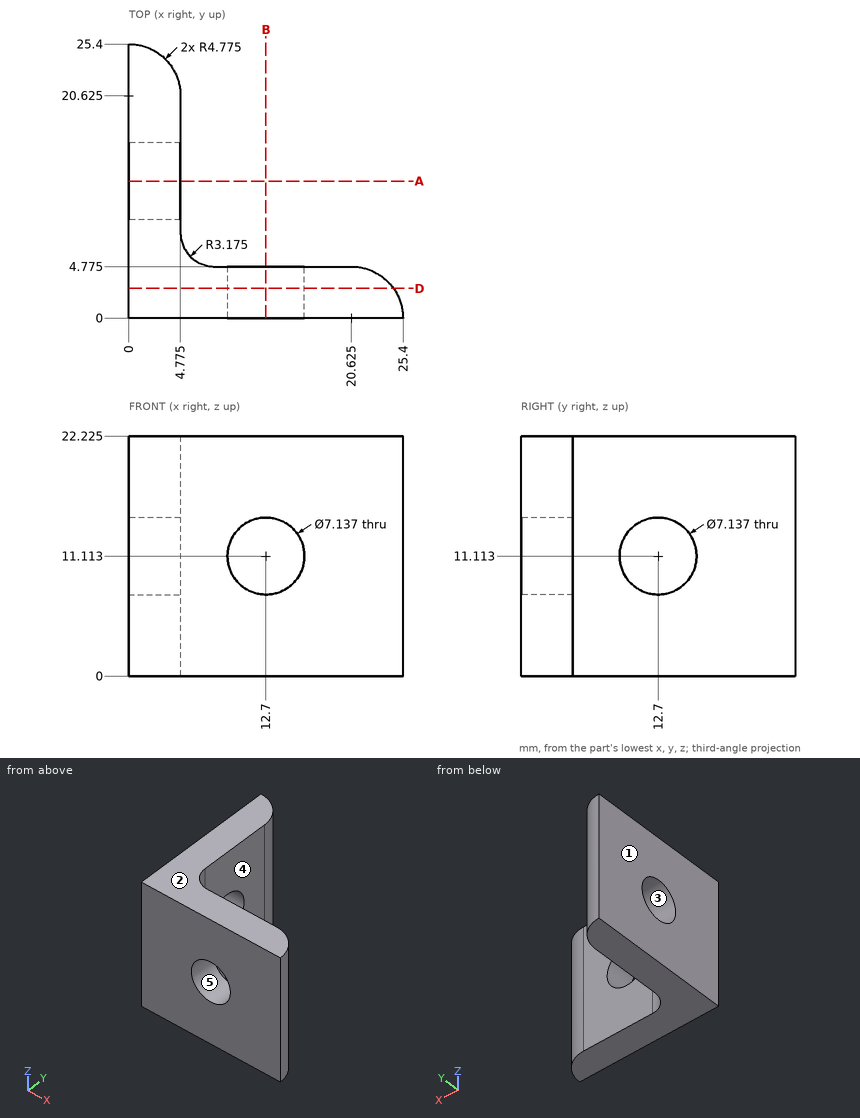
The drawing under review shows one solid part. Ordinate dimensions are in mm from its lowest x, y, z. A direction names the side the tool comes from. Round coordinates to 2 decimals unless told otherwise and drop trailing zeros. Loops run counter-clockwise (first coordinate to the right, second up) from the corner with the lowest first, then second, coordinate; pieces in that order, holes last. Notation, with made-up numbers: (16, -16) - (27, -16) arc R26 ccw to (27, 2) - close; hole circle Ø8 at (83, -19.5). An arc over 180 degrees is marked (long way). Use a Markdown table: item, result. Add a question column.
Q1. Add section D-D (y = 2.75). State the section outline as (x, z) points (1 decimal), plus the area to 3 significant figures.
Q2. The part is to be moulded in two halves that separate along Z. For the marked faces 1, 2 and 3, say which applies: pulls with the +Z half, pulls with the -Z half, needs draft (parallel to the pull), parting line crosses it, or undercut.
Q3. Machinability: for the marked faces 4 and 5, which of the approach directions +Z, -Z, +X, -X, +Y, -Y give a long, thin tool a straight path to every point of the face, cutting with its end or side? Answer none if there is none.
Q4. Add section A-A (y = 12.7). State the section outline as (x, z) points (1 decimal).
Q5. For probe 1 along Y at (x, z) = (18, 9.75) (1 decimal); probe 2 along Z at (x, y) = (3.7, 12.7) (1 decimal), list the stretches that pass through material, from the lowest coordinate up.
Q6. Insertion check: pin 1 Ø4.5 at (y, z) = (12.7, 11.11) entering from +X; pin 2 Ø10 at (x, z) = (16, 9.5) entering from +Y (1 decimal); pin 3 Ø5 at (y, z) = (8.5, 17) entering from +X (1 decimal); pin 4 Ø8 at (y, z) = (15.5, 14) entering from +X (1 decimal). Each pin has a flat end and moves straight along its axis. Give the tip position at first contact, or say it passes through.
Worked answers:
| question | item | result |
|---|---|---|
| 1 | outline | (0, 0) - (24.5, 0) - (24.5, 22.2) - (0, 22.2) - close; hole circle Ø7.1 at (12.7, 11.1) |
| 1 | area | 505 mm² |
| 2 | face 1 | needs draft |
| 2 | face 2 | pulls with the +Z half |
| 2 | face 3 | undercut |
| 3 | face 4 | +Z, -Z, +X, +Y |
| 3 | face 5 | +Y, -Y |
| 4 | outline | (0, 0) - (4.8, 0) - (4.8, 7.5) - (0, 7.5) - close; (0, 14.7) - (4.8, 14.7) - (4.8, 22.2) - (0, 22.2) - close |
| 5 | probe 1 | 0 to 4.8 |
| 5 | probe 2 | 0 to 7.5, 14.7 to 22.2 |
| 6 | pin 1 | through |
| 6 | pin 2 | y = 4.8 |
| 6 | pin 3 | x = 5.4 |
| 6 | pin 4 | x = 4.8 |
